from build123d import *

# Parameters (mm, degrees)
CROQUIS1_W              = 84
CROQUIS1_H              = 64
SALIENTE_EXTRUIR1_DEPTH = 3
CROQUIS2_W              = 75.8
CROQUIS2_H              = 55.8
CROQUIS2_W_2            = 69.8
CROQUIS2_H_2            = 49.8
SALIENTE_EXTRUIR2_DEPTH = 3
CROQUIS3_R              = 2.5
CORTAR_EXTRUIR1_DEPTH   = 7


with BuildPart() as part:
    # Croquis1 → Saliente-Extruir1 (new body)
    with BuildSketch(Plane(origin=(0, 0, 0), x_dir=(1, 0, 0), z_dir=(0, 1, 0))):
        with Locations((42, 32)):
            Rectangle(CROQUIS1_W, CROQUIS1_H)
    extrude(amount=SALIENTE_EXTRUIR1_DEPTH)

    # Croquis2 → Saliente-Extruir2 (add)
    with BuildSketch(Plane(origin=(0, 3, 0), x_dir=(1, 0, 0), z_dir=(0, 1, 0))):
        with Locations((42, 32)):
            Rectangle(CROQUIS2_W, CROQUIS2_H)
        with Locations((42, 32)):
            Rectangle(CROQUIS2_W_2, CROQUIS2_H_2, mode=Mode.SUBTRACT)
    extrude(amount=SALIENTE_EXTRUIR2_DEPTH)

    # Croquis3 → Cortar-Extruir1 (cut, through all)
    with BuildSketch(Plane.XZ):
        with Locations((42, -32)):
            Circle(CROQUIS3_R)
        with Locations((10, -10)):
            Circle(CROQUIS3_R)
        with Locations((74, -10)):
            Circle(CROQUIS3_R)
        with Locations((74, -54)):
            Circle(CROQUIS3_R)
        with Locations((10, -54)):
            Circle(CROQUIS3_R)
    extrude(amount=-CORTAR_EXTRUIR1_DEPTH, mode=Mode.SUBTRACT)


solid = part.part
The listing builds one solid part. Answer for the finished solid, in the listing's coordinates (mm). A direction names the side the tool comes from. Coordinates: 2 decimals unless noted, no trailing zeros. Loops run counter-clockwise (first coordinate to the right, second up) from the corner with the lowest first, then second, coordinate; pieces in that order, holes last. Notation, with made-up numbers: (-4.75, 54) -> (34.25, 54) arc R23 ccw to (34.25, 72) -> close; hole circle Ø4 at (78, 86). An arc over 180 degrees is marked (long way). Answer in a Markdown table with one row per item. Add a question column.
1. The part is cut by section D-D, the plane z = -32. Write down the section's boundary in (x, y), then the cut area to 3 significant figures.
2. The part is cut by section B-B, the plane z = -10. Write down the section's boundary in (x, y).
3. Determine the mould class of faces 1 (the cylindrical face through (71.5, 1.5, -53.9)), 2 (the flat face through (79.9, 4, -32)), 3 (the flat face through (41, 1, 0)), 4 (the flat face through (0, 1, -32)) for opening direction X: +X half, -X half, draft (parallel to the pull), parting line (faces both ways), or undercut.
4. The part is cut by section C-C, the plane y = 1.4. Write down the section's boundary in (x, z), then the cut area to 3 significant figures.
5. Consider line 1 (Z direction, x = 10, y = 1.05); line 2 (Z direction, x = 42, y = 1); line 3 (Z direction, x = 38, y = 4.8). Determine where each line is inside the solid, lowest interval first. Write a range as [from, to].
6. For faces 5 (the flat face through (4.1, 4, -32)), 6 (the flat face through (42, 4, -7.1)), 7 (the flat face through (41, 4, -4.1)), determine the directions among +Z, -Z, +X, -X, +Y, -Y from which every point of the face is accessible in a straight line to the end or side of a thin tool.
7. The part is cut by section A-A, the plane x = 10. Write down the section's boundary in (y, z).
8. Flat-ended cylindrical pins translate along their axes: P1, Ø3.5, axis at y = 5, z = -20, coming from the +X side; P2, Ø5, axis at x = 25, z = -7.5, coming from the +Y side; P3, Ø0.9, axis at x = 56.5, y = 4.5, coming from the +Z side; P4, Ø2.5, axis at y = 5, z = -20, coming from the -X side. Find the tip coordinate at first contact, or state that the pin passes through.
Answer below:
| question | item | result |
|---|---|---|
| 1 | outline | (0, 0) -> (39.5, 0) -> (39.5, 3) -> (7.1, 3) -> (7.1, 6) -> (4.1, 6) -> (4.1, 3) -> (0, 3) -> close; (44.5, 0) -> (84, 0) -> (84, 3) -> (79.9, 3) -> (79.9, 6) -> (76.9, 6) -> (76.9, 3) -> (44.5, 3) -> close |
| 1 | area | 255 mm2 |
| 2 | outline | (0, 0) -> (7.5, 0) -> (7.5, 3) -> (7.1, 3) -> (7.1, 6) -> (4.1, 6) -> (4.1, 3) -> (0, 3) -> close; (12.5, 0) -> (71.5, 0) -> (71.5, 3) -> (12.5, 3) -> close; (76.5, 0) -> (84, 0) -> (84, 3) -> (79.9, 3) -> (79.9, 6) -> (76.9, 6) -> (76.9, 3) -> (76.5, 3) -> close |
| 3 | face 1 | undercut |
| 3 | face 2 | +X half |
| 3 | face 3 | draft |
| 3 | face 4 | -X half |
| 4 | outline | (0, -64) -> (84, -64) -> (84, 0) -> (0, 0) -> close; hole circle Ø5 at (10, -54); hole circle Ø5 at (10, -10); hole circle Ø5 at (42, -32); hole circle Ø5 at (74, -54); hole circle Ø5 at (74, -10) |
| 4 | area | 5,280 mm2 |
| 5 | line 1 | [-64, -56.5], [-51.5, -12.5], [-7.5, 0] |
| 5 | line 2 | [-64, -34.5], [-29.5, 0] |
| 5 | line 3 | [-59.9, -56.9], [-7.1, -4.1] |
| 6 | face 5 | +Z, -Z, -X, +Y |
| 6 | face 6 | +Y |
| 6 | face 7 | +Z, +X, -X, +Y |
| 7 | outline | (0, -64) -> (3, -64) -> (3, -59.9) -> (6, -59.9) -> (6, -56.9) -> (3, -56.9) -> (3, -56.5) -> (0, -56.5) -> close; (0, -51.5) -> (3, -51.5) -> (3, -12.5) -> (0, -12.5) -> close; (0, -7.5) -> (3, -7.5) -> (3, -7.1) -> (6, -7.1) -> (6, -4.1) -> (3, -4.1) -> (3, 0) -> (0, 0) -> close |
| 8 | P1 | x = 79.9 |
| 8 | P2 | y = 6 |
| 8 | P3 | z = -4.1 |
| 8 | P4 | x = 4.1 |
